Can you work these out from the model? Positions are in its coordinate system, mm. A direction names the side the tool comes from. Coordinates: 2 decimals unless noted, no trailing zeros. Write each loop counter-clockwise with the first axis right and the second up, starting at its lowest first coordinate (ties: lowest second). Pieces come first, ordered by that corner, then holes. Notation, with made-up numbers: (-38, 11.5) -> (9, 11.5) arc R18 ccw to (9, 19.5) -> close; hole circle Ø7 at (72.25, -20). An arc over 180 degrees is marked (long way). Use one line per item in the form item = value.
```python
from build123d import *

# Parameters (mm, degrees)
F0_R     = 22
F0_R_2   = 18.5
F1_DEPTH = 8.5
F0_R_3   = 8
F2_DEPTH = 2
F3_R     = 0.5


with BuildPart() as f1:
    # F0 (on Top) → F1 (new body)
    with BuildSketch(Plane.XY):
        Circle(F0_R)
        Circle(F0_R_2, mode=Mode.SUBTRACT)
    extrude(amount=F1_DEPTH)

    # F0 (on Top) → F2 (join)
    with BuildSketch(Plane.XY):
        Circle(F0_R_2)
        Circle(F0_R_3, mode=Mode.SUBTRACT)
    extrude(amount=F2_DEPTH)

    # F3
    f3_edges = [f1.edges().sort_by_distance(p)[0] for p in [
        (-22, 0, 8.5),
        (-22, 0, 0),
        (-18.5, 0, 8.5),
    ]]
    fillet(f3_edges, radius=F3_R)


solid = f1.part
```
Q1. Thinking about a two-plate mould opening in X: for faces 3 (the flat face through (9, 0, 0)), 4 (the cylindrical face through (-1.73, -7.81, 0.99)), 5 (the cylindrical face through (-4.769, -21.477, 4.198)), which applies, released by +X, released by -X, zero draft, split by the parting line, or undercut?
Return value:
face_3 = zero draft
face_4 = undercut
face_5 = split by the parting line
Q2. Suppose I cut it at C-C (z = 6). Write out the boundary of the cut face in (x, y), then the cut area to 3 significant figures.
Return value:
outline = circle Ø44 at (0, 0); hole circle Ø37 at (0, 0)
area = 445 mm2
Q3. If I drill on line 1 (Y direction, x = 0, z = 6.2); line 2 (Z direction, x = 10.5, y = 10.5); line 3 (X direction, y = -6, z = 7.25), over which ranges is the centre line in solid material (lowest first)? Write a range as from..to.
Return value:
line_1 = -22..-18.5, 18.5..22
line_2 = 0..2
line_3 = -21.17..-17.5, 17.5..21.17
Q4. Suppose I cut it at A-A (x = 0). Write out the boundary of the cut face in (y, z).
Return value:
outline = (-22, 0.5) arc R0.5 ccw to (-21.5, 0) -> (-8, 0) -> (-8, 2) -> (-18.5, 2) -> (-18.5, 8) arc R0.5 ccw to (-19, 8.5) -> (-21.5, 8.5) arc R0.5 ccw to (-22, 8) -> close; (8, 0) -> (21.5, 0) arc R0.5 ccw to (22, 0.5) -> (22, 8) arc R0.5 ccw to (21.5, 8.5) -> (19, 8.5) arc R0.5 ccw to (18.5, 8) -> (18.5, 2) -> (8, 2) -> close
Q5. Will these pins go through, and if not, where does the flat tip stop? pin 1 (1.5 mm diameter, centred on y = -15, z = 6, fed in from -X); pin 2 (3 mm diameter, centred on y = -16.5, z = 1.5, fed in from -X); pin 3 (4 mm diameter, centred on x = -4.5, z = 1, fed in from -Y).
Return value:
pin_1 = -16.76
pin_2 = -16.09
pin_3 = -21.86
Q6. For faces 1 (the flat face through (8, -4, 2)), 2 (the flat face through (11, -16, 8.5)), which set-ups out of +Z, -Z, +X, -X, +Y, -Y let a thin tool reach every point of the face, with its end or its side?
Return value:
face_1 = +Z
face_2 = +Z, +X, -X, +Y, -Y
